Check sheet for the modelled part. Datum: model origin and axes. Units: mm. A direction names the side the tool comes from. Round coordinates to 2 decimals unless told otherwise and drop trailing zeros. Loops run counter-clockwise (first coordinate to the right, second up) from the corner with the lowest first, then second, coordinate; pieces in that order, holes last. Notation, with made-up numbers: (53.5, 62) - (92.5, 62) arc R14 cw to (92.5, 71) - close; hole circle Ø6 at (69.25, -31.5). An arc over 180 degrees is marked (long way). Return JSON: item names as keys, results as strings.
from build123d import *

# Parameters (mm, degrees)
SZKIC1_W                    = 320
SZKIC1_H                    = 380
DODANIE_WYCI_GNI_CIE1_DEPTH = 202
SZKIC2_R                    = 75.8204014
DODANIE_WYCI_GNI_CIE2_DEPTH = 16
SZKIC3_R                    = 28.051161272
DODANIE_WYCI_GNI_CIE3_DEPTH = 176
ZAOKR_GLENIE1_R             = 10


with BuildPart() as part:
    # Szkic1 → Dodanie-wyciągnięcie1 (new body)
    with BuildSketch(Plane.XY):
        with Locations((180.509851846, 381.331636977)):
            Rectangle(SZKIC1_W, SZKIC1_H)
    extrude(amount=DODANIE_WYCI_GNI_CIE1_DEPTH)

    # Szkic2 → Dodanie-wyciągnięcie2 (add)
    with BuildSketch(Plane.ZY.offset(-20.509851846)):
        with Locations(Location((101, 472.09116861, 0), (0, 0, 270))):
            Circle(SZKIC2_R)
    extrude(amount=DODANIE_WYCI_GNI_CIE2_DEPTH)

    # Szkic3 → Dodanie-wyciągnięcie3 (add)
    with BuildSketch(Plane.ZY.offset(-4.509851846)):
        with Locations(Location((101, 472.09116861, 0), (0, 0, 270))):
            Circle(SZKIC3_R)
    extrude(amount=DODANIE_WYCI_GNI_CIE3_DEPTH)

    # Dodanie-wyciągnięcie4 cone 1 section (through the dimple's axis) → Dodanie-wyciągnięcie4 (revolve)
    with BuildSketch(Plane(origin=(-171.490148154, 472.09116861, 101), x_dir=(0, 0, -1), z_dir=(0, 1, 0))):
        Polygon((0, 0), (8.316206597, 0), (0, 22.848589841), align=None)
    revolve(axis=Axis((-171.490148154, 472.09116861, 101), (-1, 0, 0)))

    # Zaokrąglenie1
    zaokr_glenie1_edges = [part.edges().sort_by_distance(p)[0] for p in [
        (20.509851846, 381.331636977, 202),
        (340.509851846, 381.331636977, 202),
        (20.509851846, 381.331636977, 0),
        (340.509851846, 381.331636977, 0),
    ]]
    fillet(zaokr_glenie1_edges, radius=ZAOKR_GLENIE1_R)


solid = part.part
Q1. Sectioned sample at A-A (y = 325). Enter the section's corners in (x, z).
Answer key:
{"outline": "(20.51, 10) arc R10 ccw to (30.51, 0) - (330.51, 0) arc R10 ccw to (340.51, 10) - (340.51, 192) arc R10 ccw to (330.51, 202) - (30.51, 202) arc R10 ccw to (20.51, 192) - close"}
Q2. Sectioned sample at D-D (y = 434.5). Enter the section's corners in (x, z), plus the area to 3 significant figures.
Answer key:
{"outline": "(4.51, 35.15) - (20.51, 35.15) - (20.51, 10) arc R10 ccw to (30.51, 0) - (330.51, 0) arc R10 ccw to (340.51, 10) - (340.51, 192) arc R10 ccw to (330.51, 202) - (30.51, 202) arc R10 ccw to (20.51, 192) - (20.51, 166.85) - (4.51, 166.85) - close", "area": "66,700 mm²"}
Q3. Tool access check on faces 1 (the face through (12.622, 527.974, 152.243)), 2 (the face through (178, 384, 202)). Record the directions out of +Z, -Z, +X, -X, +Y, -Y that give a thin tool (end or side, any length) a straight path to the whole face; none if there is none.
Answer key:
{"face 1": "-X", "face 2": "+Z, +X, -X, +Y, -Y"}
Q4. Sectioned sample at B-B (z = 146.5). Enter the section's corners in (x, y).
Answer key:
{"outline": "(4.51, 411.44) - (20.51, 411.44) - (20.51, 191.33) - (340.51, 191.33) - (340.51, 571.33) - (20.51, 571.33) - (20.51, 532.74) - (4.51, 532.74) - close"}
Q5. Sectioned sample at C-C (x = -128). Enter the section's corners in (y, z).
Answer key:
{"outline": "circle Ø56.1 at (472.09, 101)"}
Q6. Scan lines: probe 1 along X at (y, z) = (376, 90); probe 2 along X at (y, z) = (421.5, 108); probe 3 along Z at (x, y) = (0, 473.5). Record each from-to range of solid material in increasing order. Write a range as [from, to].
Answer key:
{"probe 1": "x = [20.51, 340.51]", "probe 2": "x = [4.51, 340.51]", "probe 3": "z = [72.98, 129.02]"}
